Part model, mm, in its own coordinate system. Face numbers are marked on the shaded views. A direction names the side the tool comes from. Coordinates: 2 decimals unless noted, no trailing zeros. Loops run counter-clockwise (first coordinate to the right, second up) from the corner with the lowest first, then second, coordinate; pieces in that order, holes last.
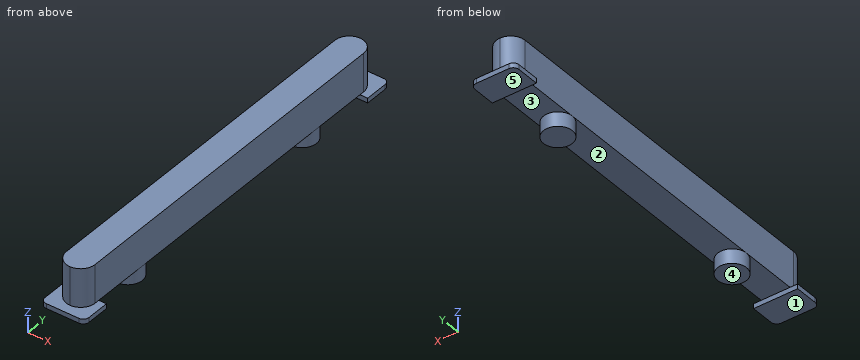
```python
from build123d import *

# Parameters (mm, degrees)
F0_W     = 1.5
F0_H     = 1
F1_DEPTH = 2
F2_DEPTH = 0.25
F3_DEPTH = 0.75
F4_R     = 0.74999
F5_R     = 0.3


# Not quite as in the source:
# - a fillet or chamfer is up to 0.001 mm smaller than in the source, because OpenCascade refuses the exact size


with BuildPart() as f1:
    # F0 (on Top) → F1 (new body)
    with BuildSketch(Plane.XY):
        with Locations((-0.75, 9.1787409857)):
            Rectangle(F0_W, F0_H)
        with BuildLine():
            Line((0, 8.6787409857), (-1.5, 8.6787409857))
            Line((-1.5, 8.6787409857), (-1.5, 5.6787409857))
            ThreePointArc((-1.5, 5.6787409857), (-0.75, 6.4287409857), (0, 5.6787409857))
            Line((0, 5.6787409857), (0, 8.6787409857))
        make_face()
        with BuildLine():
            ThreePointArc((0, 5.6787409857), (-0.75, 6.4287409857), (-1.5, 5.6787409857))
            ThreePointArc((-1.5, 5.6787409857), (-0.75, 4.9287409857), (0, 5.6787409857))
        make_face()
        with BuildLine():
            ThreePointArc((0, 5.6787409857), (-0.75, 4.9287409857), (-1.5, 5.6787409857))
            Line((-1.5, 5.6787409857), (-1.5, -6.3212590143))
            ThreePointArc((-1.5, -6.3212590143), (-0.75, -5.5712590143), (0, -6.3212590143))
            Line((0, -6.3212590143), (0, 5.6787409857))
        make_face()
        with BuildLine():
            ThreePointArc((0, -6.3212590143), (-0.75, -5.5712590143), (-1.5, -6.3212590143))
            ThreePointArc((-1.5, -6.3212590143), (-0.75, -7.0712590143), (0, -6.3212590143))
        make_face()
        with BuildLine():
            ThreePointArc((0, -6.3212590143), (-0.75, -7.0712590143), (-1.5, -6.3212590143))
            Line((-1.5, -6.3212590143), (-1.5, -9.3212590143))
            Line((-1.5, -9.3212590143), (0, -9.3212590143))
            Line((0, -9.3212590143), (0, -6.3212590143))
        make_face()
        with Locations((-0.75, -9.8212590143)):
            Rectangle(F0_W, F0_H)
    extrude(amount=F1_DEPTH)

    # F0 (on Top) → F2 (join)
    with BuildSketch(Plane.XY):
        with Locations((-0.75, -9.8212590143)):
            Rectangle(F0_W, F0_H)
        Polygon((-1.5, -10.3212590143), (-1.5, -9.3212590143), (-1.9, -9.3212590143), (-1.9, -10.8212590143), (0.4, -10.8212590143), (0.4, -9.3212590143), (0, -9.3212590143), (0, -10.3212590143), align=None)
        Polygon((-1.5, 8.6787409857), (-1.5, 9.6787409857), (0, 9.6787409857), (0, 8.6787409857), (0.4, 8.6787409857), (0.4, 10.1787409857), (-1.9, 10.1787409857), (-1.9, 8.6787409857), align=None)
        with Locations((-0.75, 9.1787409857)):
            Rectangle(F0_W, F0_H)
    extrude(amount=-F2_DEPTH)

    # F0 (on Top) → F3 (join)
    with BuildSketch(Plane.XY):
        with BuildLine():
            ThreePointArc((0, -6.3212590143), (-0.75, -5.5712590143), (-1.5, -6.3212590143))
            ThreePointArc((-1.5, -6.3212590143), (-0.75, -7.0712590143), (0, -6.3212590143))
        make_face()
        with BuildLine():
            ThreePointArc((0, 5.6787409857), (-0.75, 6.4287409857), (-1.5, 5.6787409857))
            ThreePointArc((-1.5, 5.6787409857), (-0.75, 4.9287409857), (0, 5.6787409857))
        make_face()
    extrude(amount=-F3_DEPTH)

    # F4 (radius 0.75 in the source; OpenCascade refuses exactly that, so slightly less here)
    f4_edges = [f1.edges().sort_by_distance(p)[0] for p in [
        (0, 9.678741, 1),
        (-1.5, 9.678741, 1),
        (0, -10.321259, 1),
        (-1.5, -10.321259, 1),
    ]]
    fillet(f4_edges, radius=F4_R)

    # F5
    f5_edges = [f1.edges().sort_by_distance(p)[0] for p in [
        (0.4, 10.178741, -0.125),
        (-1.9, 10.178741, -0.125),
        (0.4, -10.821259, -0.125),
        (-1.9, -10.821259, -0.125),
    ]]
    fillet(f5_edges, radius=F5_R)


solid = f1.part
```
Q1. Probe line 1 (Y direction, x = -1.55, z = -0.1); line 2 (Z direction, x = -1.45, y = 7); line 3 (X direction, y = -7.5, z = 1.1). List the from-to ranges inside material, lowest first.
Q2. Drop flat-ended pins along their axis: P1, Ø1, axis at y = -8, z = 0.5, coming from the +X side; P2, Ø0.6, axis at y = 1.5, z = 1.5, coming from the -X side; P3, Ø1.2, axis at x = -1, y = -8.5, coming from the -Z side. Give the stop position or say it passes through.
Q3. Saw through at D-D (x = -0.3). List the corners of the cut face in (y, z).
Q4. Saw through at C-C (y = -6). List the corners of the cut face in (x, z), plus the area to 3 significant figures.
Q5. Mould opens along Y. For the marked faces 1, 2 and 3 say: released by +Y, released by -Y, zero draft, split by the parting line, or undercut.
Q6. Tool access for the marked faces 4 and 5: list every direction of +Z, -Z, +X, -X, +Y, -Y with a clear straight run to the whole face (end or side of a thin tool).
Q7. Saw through at B-B (x = -1.05). List the corners of the cut face in (y, z).
Checked values:
1. line 1: y = -10.82 to -9.32, 8.68 to 10.18
1. line 2: z = 0 to 2
1. line 3: x = -1.5 to 0
2. P1: stops at x = 0
2. P2: stops at x = -1.5
2. P3: stops at z = 0
3. outline: (-10.82, -0.25) - (-9.32, -0.25) - (-9.32, 0) - (-6.92, 0) - (-6.92, -0.75) - (-5.72, -0.75) - (-5.72, 0) - (5.08, 0) - (5.08, -0.75) - (6.28, -0.75) - (6.28, 0) - (8.68, 0) - (8.68, -0.25) - (10.18, -0.25) - (10.18, 0) - (9.53, 0) - (9.53, 2) - (-10.17, 2) - (-10.17, 0) - (-10.82, 0) - close
4. outline: (-1.5, 0) - (-1.43, 0) - (-1.43, -0.75) - (-0.07, -0.75) - (-0.07, 0) - (0, 0) - (0, 2) - (-1.5, 2) - close
4. area: 4.02 mm2
5. face 1: zero draft
5. face 2: undercut
5. face 3: undercut
6. face 4: -Z, +X, -X, +Y, -Y
6. face 5: -Z, +X, -X, +Y
7. outline: (-10.82, -0.25) - (-9.32, -0.25) - (-9.32, 0) - (-7.01, 0) - (-7.01, -0.75) - (-5.63, -0.75) - (-5.63, 0) - (4.99, 0) - (4.99, -0.75) - (6.37, -0.75) - (6.37, 0) - (8.68, 0) - (8.68, -0.25) - (10.18, -0.25) - (10.18, 0) - (9.62, 0) - (9.62, 2) - (-10.26, 2) - (-10.26, 0) - (-10.82, 0) - close
